```python
from build123d import *

# Parameters (mm, degrees)
SKETCH1_W            = 49.332
SKETCH1_H            = 50
SKETCH1_W_2          = 4
SKETCH1_H_2          = 40
BOSS_EXTRUDE1_DEPTH  = 4
SKETCH2_W            = 4.134
SKETCH2_H            = 50
BOSS_EXTRUDE2_DEPTH  = 6
SKETCH8_W            = 4.134
SKETCH8_H            = 50
BOSS_EXTRUDE6_DEPTH  = 6
SKETCH9_W            = 26.398
SKETCH9_H            = 19.7
BOSS_EXTRUDE7_DEPTH  = 6
SKETCH10_W           = 26.398
SKETCH10_H           = 5
BOSS_EXTRUDE8_DEPTH  = 6
SKETCH11_W           = 5
SKETCH11_H           = 5
CUT_EXTRUDE1_DEPTH   = 7
FILLET9_R            = 1.5
FILLET10_R           = 1.5
FILLET13_R           = 1.5
FILLET14_R           = 1.5
FILLET15_R           = 1.5
SKETCH12_W           = 26.398
SKETCH12_H           = 25.3
CUT_EXTRUDE2_DEPTH   = 1
SKETCH13_W           = 26.398
SKETCH13_H           = 2.7
BOSS_EXTRUDE10_DEPTH = 1.5
FILLET18_R           = 1.5
FILLET19_R           = 1.5


with BuildPart() as part:
    # Sketch1 → Boss-Extrude1 (new body)
    with BuildSketch(Plane(origin=(0, 0, 0), x_dir=(1, 0, 0), z_dir=(0, 1, 0))):
        with Locations((7.133329328, 13.494184872)):
            Rectangle(SKETCH1_W, SKETCH1_H)
        with Locations((26.466329328, 13.494184872)):
            Rectangle(SKETCH1_W_2, SKETCH1_H_2, mode=Mode.SUBTRACT)
        with Locations((-12.199670672, 13.494184872)):
            Rectangle(SKETCH1_W_2, SKETCH1_H_2, mode=Mode.SUBTRACT)
    extrude(amount=BOSS_EXTRUDE1_DEPTH)

    # Sketch2 → Boss-Extrude2 (add)
    with BuildSketch(Plane(origin=(0, 4, 0), x_dir=(1, 0, 0), z_dir=(0, 1, 0))):
        with Locations((-8.132670672, 13.494184872)):
            Rectangle(SKETCH2_W, SKETCH2_H)
    extrude(amount=BOSS_EXTRUDE2_DEPTH)

    # Sketch8 → Boss-Extrude6 (add)
    with BuildSketch(Plane(origin=(0, 4, 0), x_dir=(1, 0, 0), z_dir=(0, 1, 0))):
        with Locations((22.399329328, 13.494184872)):
            Rectangle(SKETCH8_W, SKETCH8_H)
    extrude(amount=BOSS_EXTRUDE6_DEPTH)

    # Sketch9 → Boss-Extrude7 (add)
    with BuildSketch(Plane(origin=(0, 4, 0), x_dir=(1, 0, 0), z_dir=(0, 1, 0))):
        with Locations((7.133329328, 28.644184872)):
            Rectangle(SKETCH9_W, SKETCH9_H)
    extrude(amount=BOSS_EXTRUDE7_DEPTH)

    # Sketch10 → Boss-Extrude8 (add)
    with BuildSketch(Plane(origin=(0, 4, 0), x_dir=(1, 0, 0), z_dir=(0, 1, 0))):
        with Locations((7.133329328, -9.005815128)):
            Rectangle(SKETCH10_W, SKETCH10_H)
    extrude(amount=BOSS_EXTRUDE8_DEPTH)

    # Sketch11 → Cut-Extrude1 (cut)
    with BuildSketch(Plane(origin=(0, 10, 0), x_dir=(1, 0, 0), z_dir=(0, 1, 0))):
        with Locations((7.134329328, -9.005815128)):
            Rectangle(SKETCH11_W, SKETCH11_H)
    extrude(amount=-CUT_EXTRUDE1_DEPTH, mode=Mode.SUBTRACT)

    # Fillet9
    fillet9_edges = [part.edges().sort_by_distance(p)[0] for p in [
        (-10.199670672, 4, 9.005815128),
    ]]
    fillet(fillet9_edges, radius=FILLET9_R)

    # Fillet10
    fillet10_edges = [part.edges().sort_by_distance(p)[0] for p in [
        (-10.199670672, 4, -35.994184872),
    ]]
    fillet(fillet10_edges, radius=FILLET10_R)

    # Fillet13
    fillet13_edges = [part.edges().sort_by_distance(p)[0] for p in [
        (24.466329328, 4, -35.994184872),
    ]]
    fillet(fillet13_edges, radius=FILLET13_R)

    # Fillet14
    fillet14_edges = [part.edges().sort_by_distance(p)[0] for p in [
        (24.466329328, 4, 9.005815128),
    ]]
    fillet(fillet14_edges, radius=FILLET14_R)

    # Fillet15
    fillet15_edges = [part.edges().sort_by_distance(p)[0] for p in [
        (4.634329328, 10, 9.005815128),
        (9.634329328, 10, 9.005815128),
        (31.799329328, 4, -13.494184872),
        (-10.199670672, 10, -13.494184872),
        (-17.532670672, 4, -13.494184872),
        (31.799329328, 0, -13.494184872),
        (-17.532670672, 0, -13.494184872),
        (24.466329328, 10, -13.494184872),
    ]]
    fillet(fillet15_edges, radius=FILLET15_R)

    # Sketch12 → Cut-Extrude2 (cut)
    with BuildSketch(Plane(origin=(0, 4, 0), x_dir=(1, 0, 0), z_dir=(0, 1, 0))):
        with Locations((7.133329328, 6.144184872)):
            Rectangle(SKETCH12_W, SKETCH12_H)
    extrude(amount=-CUT_EXTRUDE2_DEPTH, mode=Mode.SUBTRACT)

    # Sketch13 → Boss-Extrude10 (add)
    with BuildSketch(Plane(origin=(0, 3, 0), x_dir=(1, 0, 0), z_dir=(0, 1, 0))):
        with Locations((7.133329328, 1.744184872)):
            Rectangle(SKETCH13_W, SKETCH13_H)
    extrude(amount=BOSS_EXTRUDE10_DEPTH)

    # Fillet18
    fillet18_edges = [part.edges().sort_by_distance(p)[0] for p in [
        (4.634329328, 3, 9.005815128),
    ]]
    fillet(fillet18_edges, radius=FILLET18_R)

    # Fillet19
    fillet19_edges = [part.edges().sort_by_distance(p)[0] for p in [
        (9.634329328, 3, 9.005815128),
    ]]
    fillet(fillet19_edges, radius=FILLET19_R)


solid = part.part
```
Build history of the part. All positions in model axes, mm. A direction names the side the tool comes from. Coordinates: 2 decimals unless noted, no trailing zeros. Order: outer loops, then holes, each group sorted by start corner. A loop starts at its lowest first (then second) coordinate and runs counter-clockwise, first axis right, second up. Notation, with made-up numbers: (-24, 6.5) -> (15, 6.5) arc R11 cw to (15, 13.5) -> close; hole circle Ø8 at (13, 59.25). An arc over 180 degrees is marked (long way). Answer in a Markdown table with one row per item. Add a question column.
Q1. Wall check: line 1 along X through (y, z) = (2.5, 4); line 2 along Z through (x, y) = (12, 4.25); line 3 along Z through (x, y) = (3.5, 5). Give the ranges that are in metal, low to high. Write a range as [from, to].
Q2. Mould opens along Z. For faces 1 (the face through (6.8, 2.7, 11.506)), 2 (the face through (-10.2, 4, -13)), 3 (the face through (-9.77, 9.55, -13.84)) say: +Z half, -Z half, draft (parallel to the pull), parting line (faces both ways), or undercut.
Q3. Band-saw the part on A-A, the plane z = -21. List the corners of the cut face in (x, y), then the cut area to 3 significant figures.
Q4. Drop flat-ended pins along their axis: pin 1 (2 mm diameter, centred on y = 1, z = -14, fed in from -X); pin 2 (2 mm diameter, centred on y = 5.5, z = 8.5, fed in from +X); pin 3 (2 mm diameter, centred on y = 6.5, z = -30.5, fed in from +X); pin 4 (1 mm diameter, centred on x = 5.5, y = 5.5, fed in from +Z). Give the stop position or say it passes through.
Q5. Which spindle directions (+Z, -Z, +X, -X, +Y, -Y) get a long thin tool onto all of the face, cutting with end or side? Do faces 4 (the face through (24.917, 4.428, -36.029)), 5 (the face through (-15, 4, -14)), 6 (the face through (-6.066, 6, -6)), 7 (the face through (9.634, 7, 9)), 8 (the face through (-12, 2, 6.506)). Say none if no direction does.
Q6. Band-saw the part on B-B, the plane y = 7.75. List the corners of the cut face in (x, z), then the cut area to 3 significant figures.
Q7. Band-saw the part on C-C, the plane x = 16.5. List the corners of the cut face in (y, z), then the cut area to 3 significant figures.
Q8. Band-saw the part on D-D, the plane z = -10.5. List the corners of the cut face in (x, y), then the cut area to 3 significant figures.
Answers follow:
| question | item | result |
|---|---|---|
| 1 | line 1 | [-17.53, -14.2], [-10.2, 24.47], [28.47, 31.8] |
| 1 | line 2 | [-38.49, -18.79], [-3.09, -0.39], [6.51, 11.51] |
| 1 | line 3 | [-38.49, -18.79], [6.51, 11.51] |
| 2 | face 1 | +Z half |
| 2 | face 2 | undercut |
| 2 | face 3 | draft |
| 3 | outline | (-17.53, 1.5) arc R1.5 ccw to (-16.03, 0) -> (-14.2, 0) -> (-14.2, 4) -> (-16.03, 4) arc R1.5 ccw to (-17.53, 2.5) -> close; (-10.2, 0) -> (24.47, 0) -> (24.47, 8.5) arc R1.5 ccw to (22.97, 10) -> (-8.7, 10) arc R1.5 ccw to (-10.2, 8.5) -> close; (28.47, 0) -> (30.3, 0) arc R1.5 ccw to (31.8, 1.5) -> (31.8, 2.5) arc R1.5 ccw to (30.3, 4) -> (28.47, 4) -> close |
| 3 | area | 370 mm^2 |
| 4 | pin 1 | x = -17.53 |
| 4 | pin 2 | x = 24.85 |
| 4 | pin 3 | x = 24.47 |
| 4 | pin 4 | z = -18.79 |
| 5 | face 4 | +Z, -Z, +X, +Y |
| 5 | face 5 | +Z, -Z, -X, +Y |
| 5 | face 6 | +Y |
| 5 | face 7 | +Z, +Y |
| 5 | face 8 | +Y, -Y |
| 6 | outline | (-10.2, -38.49) -> (24.47, -38.49) -> (24.47, 11.51) -> (9.63, 11.51) -> (9.63, 6.51) -> (20.33, 6.51) -> (20.33, -18.79) -> (-6.07, -18.79) -> (-6.07, 6.51) -> (4.63, 6.51) -> (4.63, 11.51) -> (-10.2, 11.51) -> close |
| 6 | area | 1,040 mm^2 |
| 7 | outline | (0, -38.49) -> (10, -38.49) -> (10, -18.79) -> (3, -18.79) -> (3, -3.09) -> (4.5, -3.09) -> (4.5, -0.39) -> (3, -0.39) -> (3, 6.51) -> (10, 6.51) -> (10, 11.51) -> (0, 11.51) -> close |
| 7 | area | 327 mm^2 |
| 8 | outline | (-17.53, 1.5) arc R1.5 ccw to (-16.03, 0) -> (-14.2, 0) -> (-14.2, 4) -> (-16.03, 4) arc R1.5 ccw to (-17.53, 2.5) -> close; (-10.2, 0) -> (24.47, 0) -> (24.47, 8.5) arc R1.5 ccw to (22.97, 10) -> (20.33, 10) -> (20.33, 3) -> (-6.07, 3) -> (-6.07, 10) -> (-8.7, 10) arc R1.5 ccw to (-10.2, 8.5) -> close; (28.47, 0) -> (30.3, 0) arc R1.5 ccw to (31.8, 1.5) -> (31.8, 2.5) arc R1.5 ccw to (30.3, 4) -> (28.47, 4) -> close |
| 8 | area | 186 mm^2 |
